```python
from build123d import *

# Parameters (mm, degrees)
ESQUISSE1_R        = 1.925
ESQUISSE1_R_2      = 1.5
BOSS_EXTRU_1_DEPTH = 5


with BuildPart() as part:
    # Esquisse1 → Boss.-Extru.1 (new body)
    with BuildSketch(Plane.XY):
        with BuildLine():
            Line((13.5, -22.5), (-13.5, -22.5))
            ThreePointArc((-13.5, -22.5), (-16.328427125, -21.328427125), (-17.5, -18.5))
            Line((-17.5, -18.5), (-17.5, 5.5))
            ThreePointArc((-17.5, 5.5), (-12.52081528, 17.52081528), (-0.5, 22.5))
            Line((-0.5, 22.5), (0.5, 22.5))
            ThreePointArc((0.5, 22.5), (12.52081528, 17.52081528), (17.5, 5.5))
            Line((17.5, 5.5), (17.5, -18.5))
            ThreePointArc((17.5, -18.5), (16.328427125, -21.328427125), (13.5, -22.5))
        make_face()
        with Locations((8.5, 12.5)):
            Circle(ESQUISSE1_R, mode=Mode.SUBTRACT)
        with Locations((-8.5, 12.5)):
            Circle(ESQUISSE1_R, mode=Mode.SUBTRACT)
        with Locations((-12.8, -13.5)):
            Circle(ESQUISSE1_R_2, mode=Mode.SUBTRACT)
        with Locations((12.8, -13.5)):
            Circle(ESQUISSE1_R_2, mode=Mode.SUBTRACT)
        with BuildLine():
            Line((-6.2, -20), (6.2, -20))
            ThreePointArc((6.2, -20), (7.260660172, -19.560660172), (7.7, -18.5))
            ThreePointArc((7.7, -18.5), (7.260660172, -17.439339828), (6.2, -17))
            Line((6.2, -17), (-6.2, -17))
            ThreePointArc((-6.2, -17), (-7.260660172, -17.439339828), (-7.7, -18.5))
            ThreePointArc((-7.7, -18.5), (-7.260660172, -19.560660172), (-6.2, -20))
        make_face(mode=Mode.SUBTRACT)
        with BuildLine():
            Line((-11.5, -9.5), (11.5, -9.5))
            Line((11.5, -9.5), (11.5, -4.5))
            Line((11.5, -4.5), (14, -4.5))
            ThreePointArc((14, -4.5), (15, -3.5), (14, -2.5))
            Line((14, -2.5), (11.5, -2.5))
            Line((11.5, -2.5), (11.5, 2.5))
            Line((11.5, 2.5), (-11.5, 2.5))
            Line((-11.5, 2.5), (-11.5, -2.5))
            Line((-11.5, -2.5), (-14, -2.5))
            ThreePointArc((-14, -2.5), (-15, -3.5), (-14, -4.5))
            Line((-14, -4.5), (-11.5, -4.5))
            Line((-11.5, -4.5), (-11.5, -9.5))
        make_face(mode=Mode.SUBTRACT)
    extrude(amount=BOSS_EXTRU_1_DEPTH)


solid = part.part
```
Work out the finished part from the listing and answer in its coordinate system (mm). A direction names the side the tool comes from. Coordinates: 2 decimals unless noted, no trailing zeros. Loops run counter-clockwise (first coordinate to the right, second up) from the corner with the lowest first, then second, coordinate; pieces in that order, holes last. Notation, with made-up numbers: M 3.25,26 L 38.25,26 A16 cw 38.25,54 Z; hole C 48.25,42.5 d6. An arc over 180 degrees is marked long. Use CSV: the item, a comma, the result in double quotes. Start each with the question number.
(1) Find section C-C, the plane z = 3.2. Give the vertices of the cut face in (x, y) (3 decimals).
(2) Consider line 1 (Y direction, x = -0.5, z = 2); line 2 (Y direction, x = -8.5, z = 2.05) (3 decimals); line 3 (X direction, y = 2, z = 1.7). Determine where each line is inside the solid, lowest interval first.
(3) For faces 5 (the face through (-12.65, 17.39, 2.46)), 6 (the face through (0, -20, 2)), determine the directions among +Z, -Z, +X, -X, +Y, -Y from which every point of the face is accessible in a straight line to the end or side of a thin tool.
(4) Find section B-B, the plane x = -12.8. Give the vertices of the cut face in (y, z) (3 decimals).
(5) For a pull along X with two mould halves and no side action, classify faces 1 (the face through (0, -9.5, 2)), 2 (the face through (-11.414, -14.075, 2.465)), 3 (the face through (0, -22.5, 2)), 4 (the face through (12.39, 17.65, 2.46)) as +X half, -X half, draft (parallel to the pull), parting line (faces both ways), or undercut.
(6) Find section D-D, the plane y = -3.5. Give the vertices of the cut face in (x, z), then the cut area to 3 significant figures.
(7) Find section A-A, the plane y = -13.5. Give the vertices of the cut face in (x, z), then the cut area to 3 significant figures.
(8) Given pin 1 Ø0.8 at (x, z) = (13, 1.5) entering from +Y; pin 2 Ø1.5 at (x, z) = (2, 3.5) entering from +Y, each flat-ended and moving along its own axis, determine where each tip first touches the part or whether it passes through.
Recorded:
1,outline,"M -17.5,-18.5 A4 ccw -13.5,-22.5 L 13.5,-22.5 A4 ccw 17.5,-18.5 L 17.5,5.5 A17 ccw 0.5,22.5 L -0.5,22.5 A17 ccw -17.5,5.5 Z; hole C -12.8,-13.5 d3; hole M -14,-4.5 L -11.5,-4.5 L -11.5,-9.5 L 11.5,-9.5 L 11.5,-4.5 L 14,-4.5 A1 ccw 14,-2.5 L 11.5,-2.5 L 11.5,2.5 L -11.5,2.5 L -11.5,-2.5 L -14,-2.5 A1 ccw Z; hole C -8.5,12.5 d3.85; hole M -6.2,-20 L 6.2,-20 A1.5 ccw 6.2,-17 L -6.2,-17 A1.5 ccw Z; hole C 8.5,12.5 d3.85; hole C 12.8,-13.5 d3"
2,line 1,"y = -22.5 to -20, -17 to -9.5, 2.5 to 22.5"
2,line 2,"y = -22.5 to -9.5, 2.5 to 10.575, 14.425 to 20.5"
2,line 3,"x = -17.5 to -11.5, 11.5 to 17.5"
3,face 5,"+Z, -Z, -X, +Y"
3,face 6,"+Z, -Z"
4,outline,"M -22.5,0 L -15,0 L -15,5 L -22.5,5 Z; M -12,0 L -4.5,0 L -4.5,5 L -12,5 Z; M -2.5,0 L 17.235,0 L 17.235,5 L -2.5,5 Z"
5,face 1,"undercut"
5,face 2,"undercut"
5,face 3,"draft"
5,face 4,"+X half"
6,outline,"M -17.5,0 L -15,0 L -15,5 L -17.5,5 Z; M 15,0 L 17.5,0 L 17.5,5 L 15,5 Z"
6,area,"25.0 mm^2"
7,outline,"M -17.5,0 L -14.3,0 L -14.3,5 L -17.5,5 Z; M -11.3,0 L 11.3,0 L 11.3,5 L -11.3,5 Z; M 14.3,0 L 17.5,0 L 17.5,5 L 14.3,5 Z"
7,area,"145 mm^2"
8,pin 1,"stops at y = 17.44"
8,pin 2,"stops at y = 22.48"
